The listing builds one solid part. Answer for the finished solid, in the listing's coordinates (mm). Face numbers are marked on the shaded views. A direction names the side the tool comes from. Coordinates: 2 decimals unless noted, no trailing zeros. Write each loop counter-clockwise with the first axis right and the second up, starting at its lowest first coordinate (ties: lowest second). Pieces come first, ordered by that corner, then holes. Notation, with made-up numbers: M 50,35.25 L 89,35.25 A5 cw 89,41.25 Z; hole C -6.5,48.25 d10. An arc over 180 degrees is marked long. Answer as CSV lines item,"result".
```python
from build123d import *

# Parameters (mm, degrees)
F0_R     = 17.819114
F1_DEPTH = 25.4
F2_W     = 50.421048
F2_H     = 28.575002
F3_DEPTH = 12.7
F4_R     = 11.764815
F5_DEPTH = 25.4
F7_DEPTH = 1.524


with BuildPart() as f1:
    # F0 (on Top) → F1 (new body)
    with BuildSketch(Plane.XY):
        Circle(F0_R)
    extrude(amount=F1_DEPTH)

    # F2 (on Top) → F3 (join)
    with BuildSketch(Plane.XY):
        with Locations((-25.210524, 0)):
            Rectangle(F2_W, F2_H)
    extrude(amount=F3_DEPTH)

    # F4 (on Top) → F5 (cut)
    with BuildSketch(Plane.XY):
        Circle(F4_R)
    extrude(amount=F5_DEPTH, mode=Mode.SUBTRACT)

    # F6 (on Front) → F7 (join)
    with BuildSketch(Plane.XZ):
        Polygon((-17.237177, 21.292984), (-35.119597, 12.812662), (-17.237177, 12.259597), align=None)
    extrude(amount=F7_DEPTH)


solid = f1.part
```
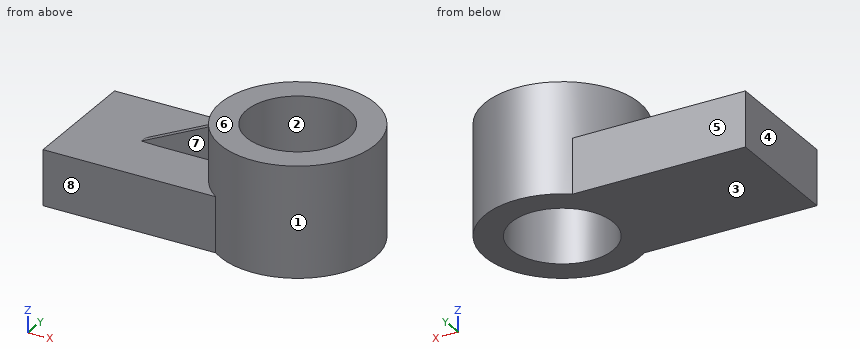
Q1. Find section C-C (z = 12). Give the vertices of the cut face in (x, y).
Output:
outline,"M -50.42,-14.29 L -10.65,-14.29 A17.82 ccw long -10.65,14.29 L -50.42,14.29 Z; hole C 0,0 d23.53"
Q2. Find section A-A (x = 0). Give the vertices of the cut face in (y, z).
Output:
outline,"M -17.82,0 L -11.76,0 L -11.76,25.4 L -17.82,25.4 Z; M 11.76,0 L 17.82,0 L 17.82,25.4 L 11.76,25.4 Z"
Q3. Straight lines are drawn through the part: line 1 (Y direction, x = 0, z = 15); line 2 (Y direction, x = -28, z = 11.25); line 3 (Y direction, x = 4, z = 7.5). For each, find the intervals that lie inside material, in ascending order.
Output:
line 1,"-17.82 to -11.76, 11.76 to 17.82"
line 2,"-14.29 to 14.29"
line 3,"-17.36 to -11.06, 11.06 to 17.36"
Q4. Flat-ended cylindrical pins translate along their axes: pin 1 Ø19 at (x, y) = (0, 0) entering from -Z; pin 2 Ø10 at (x, z) = (-4.5, 18.5) entering from -Y; pin 3 Ø6.5 at (x, z) = (-24, 15) entering from -Y; pin 4 Ø1.5 at (x, z) = (-39, 13) entering from +Y. Find the tip coordinate at first contact, or state that the pin passes through.
Output:
pin 1,"through"
pin 2,"y = -17.82"
pin 3,"y = -14.29"
pin 4,"y = 14.29"
Q5. For the marked faces 5, 6, 7 and 8, determine the directions among +Z, -Z, +X, -X, +Y, -Y from which every point of the face is accessible in a straight line to the end or side of a thin tool.
Output:
face 5,"+Z, -Z, -X, +Y"
face 6,"+Z, +X, -X, +Y, -Y"
face 7,"+Z, -X, -Y"
face 8,"+Z, -Z, -X, -Y"
Q6. Find section B-B (y = -5.5). Give the vertices of the cut face in (x, z).
Output:
outline,"M -50.42,0 L -10.4,0 L -10.4,25.4 L -16.95,25.4 L -16.95,12.7 L -50.42,12.7 Z; M 10.4,0 L 16.95,0 L 16.95,25.4 L 10.4,25.4 Z"
Q7. The mould has two halves that part along X. Classify the marked faces 1, 2, 3 and 4: pulls with the +X half, pulls with the -X half, needs draft (parallel to the pull), parting line crosses it, or undercut.
Output:
face 1,"parting line crosses it"
face 2,"undercut"
face 3,"needs draft"
face 4,"pulls with the -X half"
Q8. Find section D-D (z = 24.25). Give the vertices of the cut face in (x, y), and give its area (3 significant figures).
Output:
outline,"C 0,0 d35.64; hole C 0,0 d23.53"
area,"563 mm2"
